Work out the finished part from the listing and answer in its coordinate system (mm). A direction names the side the tool comes from. Give positions to 0.01 mm unless a question says otherwise; leave off trailing zeros. Write each loop counter-clockwise with the first axis right and the second up, starting at its lowest first coordinate (ties: lowest second). Pieces come first, ordered by that corner, then holes.
1) Given pin 1 Ø1.5 at (x, y) = (52.5, -7) entering from -Z; pin 2 Ø12 at (x, z) = (10, -31) entering from +Y; pin 3 Ø4 at (x, z) = (14, 8) entering from +Y; pin 4 Ø10 at (x, z) = (-7.5, -2) entering from +Y, each flat-ended and moving along its own axis, determine where each tip first touches the part or whether it passes through.
2) Find section A-A (y = 0). Determine the outline of the cut face in (x, z) (3 decimals), plus the area to 3 significant figures.
3) Straight lines are drawn through the part: probe 1 along X at (y, z) = (3.5, 19.5); probe 2 along X at (y, z) = (0.5, -15); probe 3 along Z at (x, y) = (35, 1.5). For each, find the intervals that lie inside material, in ascending order.
4) Find section B-B (x = 0). Determine the outline of the cut face in (y, z) (3 decimals).
5) A tool of negligible diameter and unlimited length cuts with its end or side. For faces 5 (the face through (5, -5, 0)), 6 (the face through (0, 0, -44.45)), from which of +Z, -Z, +X, -X, +Y, -Y can it reach the whole face along a straight path? Write none if from no direction.
6) Find section C-C (z = -36.5). Determine the outline of the cut face in (x, y), plus the area to 3 significant figures.
7) Determine the mould class of faces 1 (the face through (-1.38, 6.2, -21.91)), 2 (the face through (0, 0, 31.75)), 3 (the face through (-40.789, 2.39, 19.674)), 4 (the face through (41.515, 2.39, 19.674)) for opening direction X: pulls with the +X half, pulls with the -X half, needs draft (parallel to the pull), parting line crosses it, or undercut.
8) Find section D-D (z = 2). Determine the outline of the cut face in (x, y).
```python
from build123d import *

# Parameters (mm, degrees)
F0_R     = 15.875
F1_DEPTH = 31.75
F2_R     = 6.35
F3_DEPTH = 44.45
F4_R     = 4.445
F5_DEPTH = 76.2
F10_R    = 5.08


with BuildPart() as f1:
    # F0 (on Top) → F1 (new body)
    with BuildSketch(Plane.XY):
        Circle(F0_R)
    extrude(amount=F1_DEPTH)

    # F2 (on face) → F3 (join)
    with BuildSketch(Plane(origin=(0, 0, 0), x_dir=(1, 0, 0), z_dir=(0, 0, -1))):
        Circle(F2_R)
    extrude(amount=F3_DEPTH)

    # F4 (on Right) → F5 (join, symmetric)
    with BuildSketch(Plane.YZ):
        with Locations((0, 15.926162)):
            Circle(F4_R)
    extrude(amount=F5_DEPTH, both=True)

    # F6 (on Front) → F7 (revolve)
    with BuildSketch(Plane.XZ):
        with BuildLine():
            Line((-76.2, 15.926162), (-76.2, 20.371162))
            Line((-76.2, 20.371162), (-67.063941, 20.371162))
            ThreePointArc((-67.063941, 20.371162), (-78.480706, 25.826868), (-86.36, 15.926162))
            Line((-86.36, 15.926162), (-76.2, 15.926162))
        make_face()
    revolve(axis=Axis((-81.28, 0, 15.926162), (-1, 0, 0)))

    # F8 (on Front) → F9 (revolve)
    with BuildSketch(Plane.XZ):
        with BuildLine():
            ThreePointArc((86.36, 15.926162), (78.480706, 25.826868), (67.063941, 20.371162))
            Line((67.063941, 20.371162), (76.2, 20.371162))
            Line((76.2, 20.371162), (76.2, 15.926162))
            Line((76.2, 15.926162), (86.36, 15.926162))
        make_face()
    revolve(axis=Axis((81.28, 0, 15.926162), (1, 0, 0)))

    # F10
    f10_edges = [f1.edges().sort_by_distance(p)[0] for p in [
        (-15.875, 0, 31.75),
        (-15.875, 0, 0),
    ]]
    fillet(f10_edges, radius=F10_R)


solid = f1.part
```
Results:
1. pin 1: passes through
1. pin 2: stops at y = 4.93
1. pin 3: stops at y = 10.39
1. pin 4: stops at y = 14.21
2. outline: (-67.064, 11.481) - (-15.875, 11.481) - (-15.875, 5.08) arc R5.08 ccw to (-10.795, 0) - (-6.35, 0) - (-6.35, -44.45) - (6.35, -44.45) - (6.35, 0) - (10.795, 0) arc R5.08 ccw to (15.875, 5.08) - (15.875, 11.481) - (67.064, 11.481) arc R10.16 ccw (long way) to (67.064, 20.371) - (15.875, 20.371) - (15.875, 26.67) arc R5.08 ccw to (10.795, 31.75) - (-10.795, 31.75) arc R5.08 ccw to (-15.875, 26.67) - (-15.875, 20.371) - (-67.064, 20.371) arc R10.16 ccw (long way) to start
2. area: 3,100 mm2
3. probe 1: x = -85.04 to -67.36, -15.48 to 15.48, 67.36 to 85.04
3. probe 2: x = -6.33 to 6.33
3. probe 3: z = 11.74 to 20.11
4. outline: (-15.875, 5.08) arc R5.08 ccw to (-10.795, 0) - (-6.35, 0) - (-6.35, -44.45) - (6.35, -44.45) - (6.35, 0) - (10.795, 0) arc R5.08 ccw to (15.875, 5.08) - (15.875, 26.67) arc R5.08 ccw to (10.795, 31.75) - (-10.795, 31.75) arc R5.08 ccw to (-15.875, 26.67) - close
5. face 5: -Z
5. face 6: -Z, +X, -X, +Y, -Y
6. outline: circle Ø12.7 at (0, 0)
6. area: 127 mm2
7. face 1: parting line crosses it
7. face 2: needs draft
7. face 3: undercut
7. face 4: undercut
8. outline: circle Ø29.67 at (0, 0)
